Autodesk Fusion 360 part; units mm, degrees
sketch "Front View" plane through (0, 0, 0) normal (0, 0, 1) x (1, 0, 0)
  line L0 (0, 0) -> (21, 0)
  line L1 (0.6, 11) -> (20.4, 11)
  line L2 (0.6, 11) -> (0, 0)
  line L3 (20.4, 11) -> (21, 0)
  dimension "d1" = 21
  dimension "d2" = 19.8
  dimension "d3" = 11
extrude "Extrude1" add sketch "Front View" against normal blind 21
sketch "Pin Sketches" plane through (0, 0, 0) normal (0, -1, 0) x (1, 0, 0)
  line L0 (21, 0) -> (0, 0)
  line L1 (0, 0) -> (0, -21)
  line L2 (0, -21) -> (21, -21)
  line L3 (21, -21) -> (21, 0)
  line L4 (1.62, -18.88) -> (2.38, -18.88)
  line L5 (2.38, -18.88) -> (2.38, -18.12)
  line L6 (2.38, -18.12) -> (1.62, -18.12)
  line L7 (1.62, -18.12) -> (1.62, -18.88)
  line L8 (1.62, -18.88) -> (2.38, -18.88)
  line L9 (2.38, -18.88) -> (2.38, -1.5)
  line L10 (2.38, -1.5) -> (1.62, -1.5)
  line L11 (1.62, -1.5) -> (1.62, -18.88)
  dimension "d6" = 0.76
  dimension "d7" = 0.76
  dimension "d8" = 1.62
  dimension "d9" = 2.12
extrude "Extrude2" add sketch "Pin Sketches" along normal blind 5.8 contours L4 L5 L6 L7 L8 L9 L11 | L6 L9 L10 L11
Can you work these out from the model? Positions are in its coordinate system, mm. A direction names the side the tool comes from. Give positions to 0.01 mm unless a question says otherwise; leave off trailing zeros. Order: outer loops, then holes, each group sorted by start corner. A loop starts at its lowest first (then second) coordinate and runs counter-clockwise, first axis right, second up. Notation, with made-up numbers: (62, 57.25) - (83, 57.25) arc R26 ccw to (83, 91.25) - close; hole circle Ø11 at (-10.5, -11). An arc over 180 degrees is marked (long way). Use a Markdown table: item, result. Add a question column.
Q1. Please list where these lines run through material, in increasing order: line 1 along Y through (x, z) = (13, -17); line 2 along X through (y, z) = (-4, -4.5); line 3 along X through (y, z) = (0.5, -17).
Q2. If we section it at C-C on y = -3: Write out the boundary of the cut face in (x, z), plus the area to 3 significant figures.
Q3. I'm going to push flat-ended pins straight in: pin 1 (1.5 mm diameter, centred on x = 9.5, y = 3, fed in from +Z); pin 2 (6.5 mm diameter, centred on x = 7, z = -8.5, fed in from -Y); pin 3 (0.6 mm diameter, centred on x = 2, y = -4, fed in from +Z); pin 4 (5 mm diameter, centred on y = 9.5, z = -6, fed in from +X). Where does each tip first touch, or does it pass through?
Q4. On a 3-axis mill with a long thin cutter (end or side, diameter ignored), from which of +Z, -Z, +X, -X, +Y, -Y can I reach the whole of each face in a straight line? I mean faces 4 (the flat face through (0.304, 5.577, -10.353)), 5 (the flat face through (1.62, -3, -10)), 6 (the flat face through (2.38, -3, -10)). Say none if no direction works.
Q5. If we section it at A-A on z = -12: Write out the boundary of the cut face in (x, y), plus the area to 3 significant figures.
Q6. If we mould it in two halves opening along Z, with no side actions, what happens to faces 1 (the flat face through (20.696, 5.577, -10.353)), 2 (the flat face through (10, 6, 0)), 3 (the flat face through (10, 6, -21))? For each: released by +Z, released by -Z, zero draft, split by the parting line, or undercut.
Q7. If we section it at B-B on x = 2: Write out the boundary of the cut face in (y, z).
Q8. If we section it at D-D on x = 18.25: Write out the boundary of the cut face in (y, z).
Answers follow:
| question | item | result |
|---|---|---|
| 1 | line 1 | y = 0 to 11 |
| 1 | line 2 | x = 1.62 to 2.38 |
| 1 | line 3 | x = 0.03 to 20.97 |
| 2 | outline | (1.62, -18.88) - (2.38, -18.88) - (2.38, -1.5) - (1.62, -1.5) - close |
| 2 | area | 13.2 mm^2 |
| 3 | pin 1 | stops at z = 0 |
| 3 | pin 2 | stops at y = 0 |
| 3 | pin 3 | stops at z = -1.5 |
| 3 | pin 4 | stops at x = 20.62 |
| 4 | face 4 | +Z, -Z, -X, +Y |
| 4 | face 5 | +Z, -Z, -X, -Y |
| 4 | face 6 | +Z, -Z, +X, -Y |
| 5 | outline | (0, 0) - (1.62, 0) - (1.62, -5.8) - (2.38, -5.8) - (2.38, 0) - (21, 0) - (20.4, 11) - (0.6, 11) - close |
| 5 | area | 229 mm^2 |
| 6 | face 1 | zero draft |
| 6 | face 2 | released by +Z |
| 6 | face 3 | released by -Z |
| 7 | outline | (-5.8, -18.88) - (0, -18.88) - (0, -21) - (11, -21) - (11, 0) - (0, 0) - (0, -1.5) - (-5.8, -1.5) - close |
| 8 | outline | (0, -21) - (11, -21) - (11, 0) - (0, 0) - close |
